```python
from build123d import *

# Parameters (mm, degrees)
BOSS_EXTRUDE1_DEPTH = 40
FILLET1_R           = 0.5


with BuildPart() as part:
    # Sketch1 → Boss-Extrude1 (new body)
    with BuildSketch(Plane(origin=(0, 0, 0), x_dir=(-1, 0, 0), z_dir=(0, 1, 0))):
        Polygon((12.920084942, 17.782971123), (20.905136432, -6.792490393), (2.28e-07, -21.980960899), (-20.905135976, -6.792490393), (-12.920084486, 17.782971123), align=None)
    extrude(amount=BOSS_EXTRUDE1_DEPTH)

    # Fillet1
    fillet1_edges = [part.edges().sort_by_distance(p)[0] for p in [
        (10.452567874, 40, -14.386725646),
        (-10.45256833, 40, -14.386725646),
        (-16.912610687, 40, 5.495240365),
        (-2.28e-07, 40, 17.782971123),
        (-16.912610687, 0, 5.495240365),
        (-10.45256833, 0, -14.386725646),
        (10.452567874, 0, -14.386725646),
        (16.912610231, 0, 5.495240365),
        (-2.28e-07, 0, 17.782971123),
        (16.912610231, 40, 5.495240365),
    ]]
    fillet(fillet1_edges, radius=FILLET1_R)


solid = part.part
```
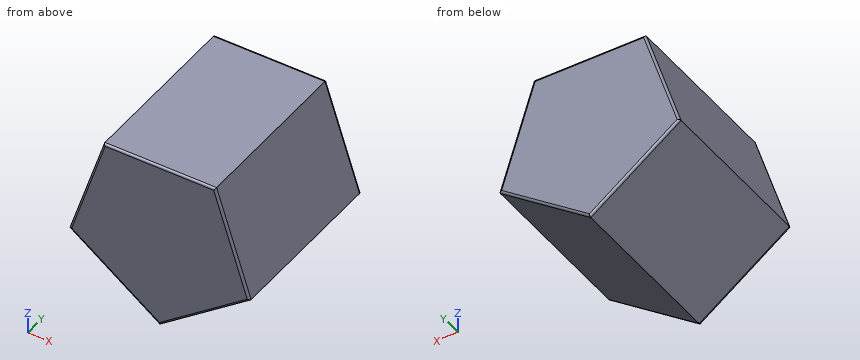
Work out the finished part from the listing and answer in its coordinate system (mm). Round coordinates to 2 decimals unless told otherwise and drop trailing zeros. Write each loop counter-clockwise with the first axis right and the second up, starting at its lowest first coordinate (ties: lowest second). Pieces come first, ordered by that corner, then holes.
1) A cutting plane is placed at A-A on y = 23. Determine the outline of the cut face in (x, z), and give its area (3 significant figures).
2) Consider probe 1 along Z at (x, y) = (1.5, 6); probe 2 along X at (y, z) = (14, -12.5); probe 3 along X at (y, z) = (2.5, 12.5). Determine where each line is inside the solid, lowest interval first.
3) Flat-ended cylindrical pins translate along their axes: P1, Ø4, axis at x = 8.5, y = 17.5, coming from the -Z side; P2, Ø6, axis at x = -4, y = 19.5, coming from the -Z side; P3, Ø5, axis at y = 4.5, z = -8, coming from the +X side. Find the tip coordinate at first contact, or state that the pin passes through.
Entries:
1. outline: (-20.91, -6.79) - (0, -21.98) - (20.91, -6.79) - (12.92, 17.78) - (-12.92, 17.78) - close
1. area: 1,150 mm2
2. probe 1: z = -20.89 to 17.78
2. probe 2: x = -13.05 to 13.05
2. probe 3: x = -14.64 to 14.64
3. P1: stops at z = -17.26
3. P2: stops at z = -21.25
3. P3: stops at x = 20.91
